Read the model definition and answer for the solid it produces. Units are mm, in the model's axes. Round coordinates to 2 decimals unless told otherwise and drop trailing zeros. Loops run counter-clockwise (first coordinate to the right, second up) from the corner with the lowest first, then second, coordinate; pieces in that order, holes last. Notation, with made-up numbers: M -0.5,53 L 43.5,53 A18 cw 43.5,65 Z; hole C 56,4.5 d4. An arc over 180 degrees is marked long. Answer as CSV lines item,"result".
```python
from build123d import *

# Parameters (mm, degrees)
SKETCH1_R                = 45.085
BASE_EXTRUDE_DEPTH       = 0.635
SKETCH2_R                = 34.925
BASE_CUT_DEPTH           = 64.762980443
SKETCH3_R                = 9.525
CORNER_EXTRUDE_DEPTH     = 0.635
SKETCH4_R                = 4.318
CORNER_CUT_DEPTH         = 64.762980443
FILLET_2_R               = 12.7
CIRPATTERN_COUNT         = 4
FILLET_2_OF_CIRPATTERN_R = 12.7


with BuildPart() as part:
    # Sketch1 → Base Extrude (new body)
    with BuildSketch(Plane(origin=(0, 0, 0), x_dir=(1, 0, 0), z_dir=(0, 1, 0))):
        with Locations(Location((0, 0, 0), (0, 0, 270))):
            Circle(SKETCH1_R)
    extrude(amount=BASE_EXTRUDE_DEPTH)

    # Sketch2 → Base Cut (cut, through all)
    with BuildSketch(Plane(origin=(0, 0.635, 0), x_dir=(1, 0, 0), z_dir=(0, 1, 0))):
        with Locations(Location((0, 0, 0), (0, 0, 270))):
            Circle(SKETCH2_R)
    extrude(amount=-BASE_CUT_DEPTH, mode=Mode.SUBTRACT)

    # Sketch3 → Corner Extrude (add)
    with BuildSketch(Plane(origin=(0, 0.635, 0), x_dir=(1, 0, 0), z_dir=(0, 1, 0))):
        with Locations((-31.87990923, 31.87990923)):
            Circle(SKETCH3_R)
    corner_extrude = extrude(amount=-CORNER_EXTRUDE_DEPTH)

    # Sketch4 → Corner Cut (cut, through all)
    with BuildSketch(Plane(origin=(0, 0.635, 0), x_dir=(1, 0, 0), z_dir=(0, 1, 0))):
        with Locations(Location((-31.87990923, 31.87990923, 0), (0, 0, 270))):
            Circle(SKETCH4_R)
    corner_cut = extrude(amount=-CORNER_CUT_DEPTH, mode=Mode.SUBTRACT)

    # Fillet 2
    fillet_2_edges = [part.edges().sort_by_distance(p)[0] for p in [
        (-24.470935923, 0.3175, -37.86595463),
        (-37.86595463, 0.3175, -24.470935923),
    ]]
    fillet(fillet_2_edges, radius=FILLET_2_R)

    # CirPattern: Corner Extrude, Corner Cut ×4 about axis
    cirpattern_axis = Axis((0, 0, 0), (0, 1, 0))
    add([corner_extrude.rotate(cirpattern_axis, i * 360 / CIRPATTERN_COUNT) for i in range(1, CIRPATTERN_COUNT)])
    add([corner_cut.rotate(cirpattern_axis, i * 360 / CIRPATTERN_COUNT) for i in range(1, CIRPATTERN_COUNT)], mode=Mode.SUBTRACT)

    # Fillet 2 of CirPattern
    fillet_2_of_cirpattern_edges = [part.edges().sort_by_distance(p)[0] for p in [
        (-37.86595463, 0.3175, 24.470935923),
        (-24.470935923, 0.3175, 37.86595463),
        (24.470935923, 0.3175, 37.86595463),
        (37.86595463, 0.3175, 24.470935923),
        (37.86595463, 0.3175, -24.470935923),
        (24.470935923, 0.3175, -37.86595463),
    ]]
    fillet(fillet_2_of_cirpattern_edges, radius=FILLET_2_OF_CIRPATTERN_R)


solid = part.part
```
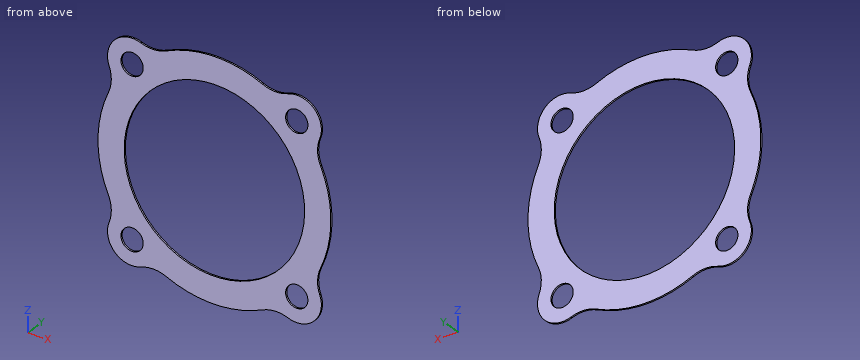
1) Find section C-C, the plane y = 0.35. Count the separate pieces of the cut face and the enclosed holes in it, then the cut area to 3 significant figures.
Evaluation:
separate pieces,"1"
enclosed holes,"5"
area,"2,970 mm^2"
2) Each of these flat-tipped pins is pushed along its axis until it touches: P1, Ø11, axis at x = 31.88, z = 31.88, coming from the +Y side (3 decimals); P2, Ø5, axis at x = -31.88, z = -31.88, coming from the +Y side. Where does it stop, or does it pass through?
Evaluation:
P1,"stops at y = 0.635"
P2,"passes through"
3) Find section B-B, the plane x = 0. Give the vertices of the cut face in (y, z) (3 decimals).
Evaluation:
outline,"M 0,-45.085 L 0.635,-45.085 L 0.635,-34.925 L 0,-34.925 Z; M 0,34.925 L 0.635,34.925 L 0.635,45.085 L 0,45.085 Z"
4) Find section A-A, the plane z = 0. Give the vertices of the cut face in (x, y) (3 decimals).
Evaluation:
outline,"M -45.085,0 L -34.925,0 L -34.925,0.635 L -45.085,0.635 Z; M 34.925,0 L 45.085,0 L 45.085,0.635 L 34.925,0.635 Z"
5) Straight lines are drawn through the part: line 1 (Z direction, x = 31, y = 0.1); line 2 (Z direction, x = 35, y = 0.5). For each, find the intervals that lie inside material, in ascending order.
Evaluation:
line 1,"z = -41.36 to -36.11, -27.65 to -16.09, 16.09 to 27.65, 36.11 to 41.36"
line 2,"z = -40.88 to -34.86, -28.89 to 28.89, 34.86 to 40.88"
